Autodesk Inventor part; units mm, degrees
ref_plane "YZ Plane" through (0, 0, 0) normal (1, 0, 0) x (0, 1, 0)
ref_plane "XZ Plane" through (0, 0, 0) normal (0, 1, 0) x (-1, 0, 0)
ref_plane "XY Plane" through (0, 0, 0) normal (0, 0, 1) x (1, 0, 0)
sketch "Sketch1" plane through (0, 0, 0) normal (0, 1, 0) x (-1, 0, 0)
  line L0 (0, 0) -> (41.148, 0)
  line L1 (41.148, 0) -> (41.148, -20.32)
  line L2 (41.148, -20.32) -> (0, -20.32)
  line L3 (0, -20.32) -> (0, 0)
  line L4 (47.498, 2.0259) -> (-5.588, 2.0259)
  line L5 (-5.588, -22.3459) -> (47.1979, -22.3459)
  circle A0 centre (45.212, -15.24) radius 2.0193
  circle A1 centre (-4.064, -15.24) radius 2.0193
  line L6 (41.148, -10.16) -> (50.3729, -10.16)
  line L7 (41.148, -13.97) -> (50.3729, -13.97)
  line L8 (41.148, -6.35) -> (50.3729, -6.35)
  line L9 (0, -10.16) -> (-8.7354, -10.16)
  line L10 (-5.588, 2.0259) -> (-5.5604, 2.0259)
  line L11 (-8.7354, -1.1491) -> (-8.7354, -19.1709)
  line L12 (-5.5604, -22.3459) -> (-5.588, -22.3459)
  line L13 (47.498, -22.3459) -> (47.1979, -22.3459)
  line L14 (50.3729, -19.1709) -> (50.3729, -1.1491)
  line L15 (47.1979, 2.0259) -> (47.498, 2.0259)
  circle A2 centre (45.212, -5.08) radius 2.0193
  circle A3 centre (-4.064, -5.08) radius 2.0193
  line L16 (-5.5604, 2.0259) -> (-8.7354, -1.1491)
  line L17 (-8.7354, -19.1709) -> (-5.5604, -22.3459)
  line L18 (47.1979, -22.3459) -> (50.3729, -19.1709)
  line L19 (50.3729, -1.1491) -> (47.1979, 2.0259)
  point P0 (41.148, -6.35)
  point P1 (41.148, -13.97)
  point P2 (-8.7354, 2.0259)
  point P3 (-8.7354, -22.3459)
  point P4 (50.3729, -22.3459)
  point P5 (50.3729, 2.0259)
  point P6 (46.7819, -6.35)
  point P7 (43.6421, -6.35)
  point P8 (43.6421, -13.97)
  point P9 (46.7819, -13.97)
  dimension "d0" = 41.148
  dimension "d1" = 20.32
  dimension "d4" = 4.0386
  dimension "d5" = 4.0386
  dimension "d6" = 3.81
  dimension "d7" = 3.81
  dimension "d16" = 5.08
  dimension "d17" = 5.08
  dimension "d18" = 4.064
  dimension "d19" = 4.064
  dimension "d20" = 3.175
  dimension "d21" = 3.175
  dimension "d22" = 3.175
  dimension "d23" = 3.175
  dimension "d24" = 3.175
  dimension "d25" = 3.175
  dimension "d26" = 3.175
  dimension "d27" = 3.175
extrude "Extrusion1" add sketch "Sketch1" along normal blind 33.02 contours L3 L9 L11 L16 L4 L19 L14 L8 A2 L1 L0 | L0 L1 L2 L3 | L3 L2 L1 L7 A0 L14 L18 L5 L17 L11 L9 | L8 A2 L14 L6 L1 | L6 L14 L7 A0 L1 | A2 L8 | L8 A2 | L7 A0 | A0 L7 | A1 | A3
extrude "Extrusion2" cut sketch "Sketch1" along normal blind 24.638 contours L7 A0 | A0 L7 | A1
extrude "Extrusion3" cut sketch "Sketch1" along normal blind 29.845 contours L0 L1 L2 L3
extrude "Extrusion4" cut sketch "Sketch1" along normal up to surface (24.638 mm away) contours L8 A2 L14 L6 L1 | L6 L14 L7 A0 L1 | A2 L8 | L8 A2 | A3
properties part number "Servo Mount and Screw Hole Test"
Geometry check sheet. Reference: the model listing, model coordinates, mm. A direction names the side the tool comes from. Give positions to 0.01 mm unless a question says otherwise; leave off trailing zeros. Order: outer loops, then holes, each group sorted by start corner. A loop starts at its lowest first (then second) coordinate and runs counter-clockwise, first axis right, second up.
1. Sectioned sample at D-D (z = -7.75). Record the boundary of the cut face in (x, y) (3 decimals).
Completed:
outline: (-50.373, 24.638) - (-41.148, 24.638) - (-41.148, 29.845) - (0, 29.845) - (0, 0) - (8.735, 0) - (8.735, 33.02) - (-50.373, 33.02) - close
2. Sectioned sample at C-C (z = -15.24). Record the boundary of the cut face in (x, y) (3 decimals), then the cut area to 3 significant figures.
Completed:
outline: (-50.373, 0) - (-47.231, 0) - (-47.231, 24.638) - (-43.193, 24.638) - (-43.193, 0) - (-41.148, 0) - (-41.148, 29.845) - (0, 29.845) - (0, 0) - (2.045, 0) - (2.045, 24.638) - (6.083, 24.638) - (6.083, 0) - (8.735, 0) - (8.735, 33.02) - (-50.373, 33.02) - close
area: 525 mm2
3. Scan lines: line 1 (Z direction, x = -30, y = 6); line 2 (Z direction, x = 5, y = 13.5); line 3 (X direction, y = 19.5, z = -16). Record each from-to range of solid material in increasing order.
Completed:
line 1: z = -22.35 to -20.32, 0 to 2.03
line 2: z = -22.35 to -17.03, -13.45 to -6.87, -3.29 to 2.03
line 3: x = -50.37 to -47.08, -43.34 to -41.15, 0 to 2.19, 5.93 to 8.74
4. Depth check by flat-ended pin: pin 1 (3 mm diameter, centred on x = -24.5, z = -18, fed in from -Y) (3 decimals); pin 2 (7.5 mm diameter, centred on x = -45, z = -10, fed in from -Y); pin 3 (1.1 mm diameter, centred on x = -49, y = 7, fed in from +Z). Enter the tip coordinate at first touch or a pass-through.
Completed:
pin 1: stops at y = 29.845
pin 2: stops at y = 24.64
pin 3: stops at z = 0.77
5. Draft check along X on faces 4 (the face through (7.126, 16.279, 0.461)), 5 (the face through (-20, 33.02, -10)), 6 (the face through (-48.808, 16.279, 0.416)), 7 (the face through (-20, 29.845, -10)). Enter one of: pulls with the +X half, pulls with the -X half, needs draft (parallel to the pull), parting line crosses it, or undercut.
Completed:
face 4: pulls with the +X half
face 5: needs draft
face 6: pulls with the -X half
face 7: undercut
6. Access from +Z, -Z, +X, -X, +Y, -Y to the whole of each face (thin tool, end or side, straight path). Record for faces 1 (the face through (-21, 16, 2.026)), 2 (the face through (4, 24.638, -15)), 3 (the face through (-49, 12, -6.35)).
Completed:
face 1: +Z, +X, -X, +Y, -Y
face 2: -Y
face 3: -X, -Y
7. Sectioned sample at A-A (y = 16). Record the boundary of the cut face in (x, z).
Completed:
outline: (-50.37, -19.17) - (-47.2, -22.35) - (5.56, -22.35) - (8.74, -19.17) - (8.74, -1.15) - (5.56, 2.03) - (-47.2, 2.03) - (-50.37, -1.15) - (-50.37, -6.35) - (-46.78, -6.35) arc R2.02 cw (long way) to (-43.64, -6.35) - (-41.15, -6.35) - (-41.15, 0) - (0, 0) - (0, -20.32) - (-41.15, -20.32) - (-41.15, -13.97) - (-43.64, -13.97) arc R2.02 cw (long way) to (-46.78, -13.97) - (-50.37, -13.97) - close; hole circle Ø4.04 at (4.06, -15.24); hole circle Ø4.04 at (4.06, -5.08)
8. Sectioned sample at B-B (x = -21). Record the boundary of the cut face in (y, z) (3 decimals), then the cut area to 3 significant figures.
Completed:
outline: (0, -22.346) - (33.02, -22.346) - (33.02, 2.026) - (0, 2.026) - (0, 0) - (29.845, 0) - (29.845, -20.32) - (0, -20.32) - close
area: 198 mm2
